Source: three-view drawing plus pictorial views. Frame: mm from the lowest corner of the part. A direction names the side the tool comes from. Give positions to 0.01 mm unless a question says otherwise; leave off trailing zeros. Loops run counter-clockwise (first coordinate to the right, second up) from the corner with the lowest first, then second, coordinate; pieces in that order, holes last. Notation, with made-up numbers: (-28, 78.5) - (-1, 78.5) arc R18 ccw to (-1, 109.5) - close; hole circle Ø6 at (-29, 60). An arc over 180 degrees is marked (long way). Answer in a Markdown table with one row per item.
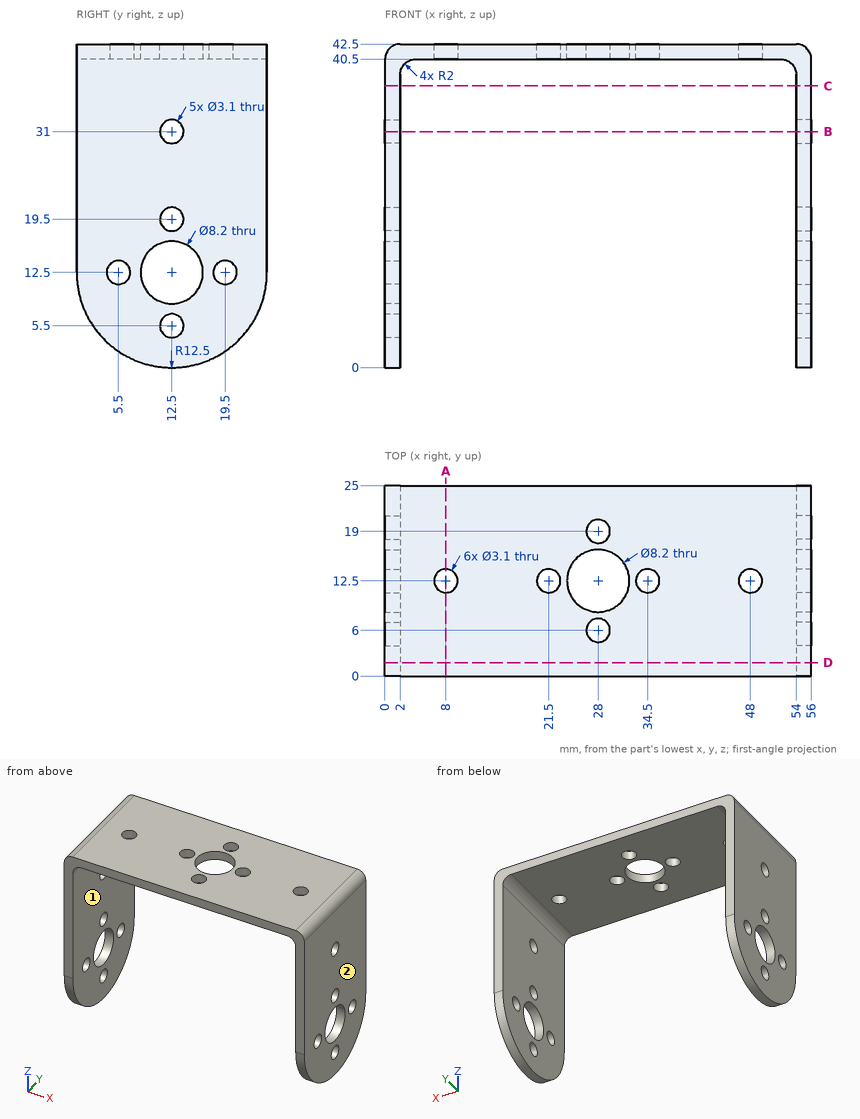
Q1. Cut plane B-B (z = 31). Output: boundary loops of the cut face in (x, y).
Check values:
| item | result |
|---|---|
| outline | (0, 0) - (2, 0) - (2, 10.95) - (0, 10.95) - close; (0, 14.05) - (2, 14.05) - (2, 25) - (0, 25) - close; (54, 0) - (56, 0) - (56, 10.95) - (54, 10.95) - close; (54, 14.05) - (56, 14.05) - (56, 25) - (54, 25) - close |
Q2. Cut plane A-A (x = 8). Output: boundary loops of the cut face in (y, z).
Check values:
| item | result |
|---|---|
| outline | (0, 40.5) - (10.95, 40.5) - (10.95, 42.5) - (0, 42.5) - close; (14.05, 40.5) - (25, 40.5) - (25, 42.5) - (14.05, 42.5) - close |
Q3. Cut plane D-D (y = 1.75). Output: boundary loops of the cut face in (x, z), and give its area (3 significant figures).
Check values:
| item | result |
|---|---|
| outline | (0, 6.12) - (2, 6.12) - (2, 38.5) arc R2 cw to (4, 40.5) - (52, 40.5) arc R2 cw to (54, 38.5) - (54, 6.12) - (56, 6.12) - (56, 40.5) arc R2 ccw to (54, 42.5) - (2, 42.5) arc R2 ccw to (0, 40.5) - close |
| area | 250 mm² |
Q4. Cut plane C-C (z = 37). Output: boundary loops of the cut face in (x, y).
Check values:
| item | result |
|---|---|
| outline | (0, 0) - (2, 0) - (2, 25) - (0, 25) - close; (54, 0) - (56, 0) - (56, 25) - (54, 25) - close |
Q5. Material intervals for line 1 along Y through (x, z) = (1.3, 12.5); line 2 along Y through (x, z) = (55, 31); line 3 along X through (y, z) = (21, 11), sorted ascending.
Check values:
| item | result |
|---|---|
| line 1 | 0 to 3.95, 7.05 to 8.4, 16.6 to 17.95, 21.05 to 25 |
| line 2 | 0 to 10.95, 14.05 to 25 |
| line 3 | 0 to 2, 54 to 56 |
Q6. First-contact query: pin 1 (3 mm diameter, centred on x = 34.5, y = 12.5, fed in from +Z); pin 2 (10.5 mm diameter, centred on x = 28, y = 12.5, fed in from -Z). Flat tips, straight axial feed; report the tip coordinate or a pass-through.
Check values:
| item | result |
|---|---|
| pin 1 | through |
| pin 2 | z = 40.5 |
Q7. Reachability of the marked faces 1 and 2 from +Z, -Z, +X, -X, +Y, -Y: full face, straight path, thin tool, end or side. Return the list, or none.
Check values:
| item | result |
|---|---|
| face 1 | -Z, +Y, -Y |
| face 2 | +Z, -Z, +X, +Y, -Y |
